from build123d import *

# Parameters (mm, degrees)
F1_DEPTH = 32
F2_W     = 20
F2_H     = 20
F3_DEPTH = 107.25
F4_W     = 139.25
F4_H     = 10
F5_DEPTH = 150


with BuildPart() as f1:
    # F0 (on Front) → F1 (new body)
    with BuildSketch(Plane.XZ):
        with BuildLine():
            Line((50, -40), (50, 40))
            Line((50, 40), (10.506873, 40))
            ThreePointArc((10.506873, 40), (0, -8.525), (-10.506873, 40))
            Line((-10.506873, 40), (-50, 40))
            Line((-50, 40), (-50, -40))
            Line((-50, -40), (50, -40))
        make_face()
    extrude(amount=F1_DEPTH)

    # F2 (on face) → F3 (join)
    with BuildSketch(Plane(origin=(0, 0, 0), x_dir=(-1, 0, 0), z_dir=(0, 1, 0))):
        with Locations((-40, 30)):
            Rectangle(F2_W, F2_H)
        with Locations((40, 30)):
            Rectangle(F2_W, F2_H)
        with Locations((40, -30)):
            Rectangle(F2_W, F2_H)
        with Locations((-40, -30)):
            Rectangle(F2_W, F2_H)
    extrude(amount=F3_DEPTH)

    # F4 (on face) → F5 (cut)
    with BuildSketch(Plane.YZ.offset(50)):
        with Locations((37.625, -35)):
            Rectangle(F4_W, F4_H)
    extrude(amount=-F5_DEPTH, mode=Mode.SUBTRACT)


solid = f1.part
Read the model definition and answer for the solid it produces. Units are mm, in the model's axes. A direction names the side the tool comes from. Give positions to 0.01 mm unless a question says otherwise; leave off trailing zeros. Write each loop counter-clockwise with the first axis right and the second up, starting at its lowest first coordinate (ties: lowest second). Pieces come first, ordered by that corner, then holes. Notation, with made-up numbers: (75.25, 85.25) - (94.25, 85.25) arc R24 cw to (94.25, 117.25) - close; hole circle Ø6 at (65, 34.25). An arc over 180 degrees is marked (long way). Answer in a Markdown table with one row per item. Add a question column.
Item 1: Determine the mould class of faces 4 (the face through (0.965, -15.776, -8.507)), 5 (the face through (40, 53, -20)), 6 (the face through (-50, 23, 21)) for opening direction X: pulls with the +X half, pulls with the -X half, needs draft (parallel to the pull), parting line crosses it, or undercut.
Item 2: A tool of negligible diameter and unlimited length cuts with its end or side. For faces 1 (the face through (-39, 23, 40)), 2 (the face through (30, 53, 30)), 3 (the face through (-40, 53, -20)), from which of +Z, -Z, +X, -X, +Y, -Y can it reach the whole face along a straight path? Write none if from no direction.
Item 3: Find the intervals of material crossed by L1, parallel to X at y = 50, z = -26; L2, parallel to Z at x = 41.5, y = 95.5; L3, parallel to Y at x = 45, z = 11, in increasing order.
Item 4: Section A-A, the plane y = 71 is taken. Write down the section's boundary in (x, z), and give its area (3 significant figures).
Item 5: Section B-B, the plane x = 34 is taken. Write down the section's boundary in (y, z).
Item 6: A flat-ended cylindrical pin translates along its axis: P1, Ø21, axis at x = -14, z = 8.5, coming from the +Y side. Find the tip coordinate at first contact, or state that the pin passes through.
Item 7: Section D-D, the plane x = 17 is taken. Write down the section's boundary in (y, z), and give its area (3 significant figures).
Item 8: Section C-C, the plane z = 4 is taken. Write down the section's boundary in (x, y), and give its area (3 significant figures).
Recorded:
| question | item | result |
|---|---|---|
| 1 | face 4 | undercut |
| 1 | face 5 | needs draft |
| 1 | face 6 | pulls with the -X half |
| 2 | face 1 | +Z, +X, -X, +Y, -Y |
| 2 | face 2 | +Z, -Z, +Y |
| 2 | face 3 | +X, -X, +Y |
| 3 | L1 | x = -50 to -30, 30 to 50 |
| 3 | L2 | z = -30 to -20, 20 to 40 |
| 3 | L3 | y = -32 to 0 |
| 4 | outline | (-50, -30) - (-30, -30) - (-30, -20) - (-50, -20) - close; (-50, 20) - (-30, 20) - (-30, 40) - (-50, 40) - close; (30, -30) - (50, -30) - (50, -20) - (30, -20) - close; (30, 20) - (50, 20) - (50, 40) - (30, 40) - close |
| 4 | area | 1,200 mm2 |
| 5 | outline | (-32, -30) - (107.25, -30) - (107.25, -20) - (0, -20) - (0, 20) - (107.25, 20) - (107.25, 40) - (-32, 40) - close |
| 6 | P1 | stops at y = 0 |
| 7 | outline | (-32, -30) - (0, -30) - (0, -2) - (-32, -2) - close; (-32, 35.75) - (0, 35.75) - (0, 40) - (-32, 40) - close |
| 7 | area | 1,030 mm2 |
| 8 | outline | (-50, -32) - (-21.9, -32) - (-21.9, 0) - (-50, 0) - close; (21.9, -32) - (50, -32) - (50, 0) - (21.9, 0) - close |
| 8 | area | 1,800 mm2 |
